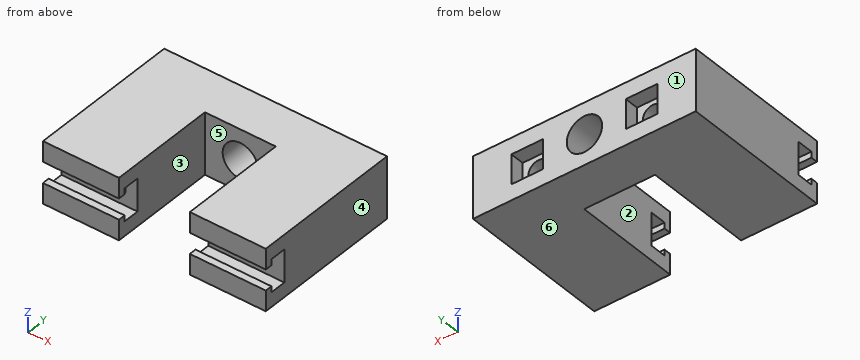
from build123d import *

# Parameters (mm, degrees)
F1_DEPTH = 11.049
F3_DEPTH = 39.9425
F4_R     = 3.175
F4_R_2   = 1.79705
F5_DEPTH = 27.307296
F4_W     = 5.678279
F4_H     = 5.299044
F6_DEPTH = 2.54


with BuildPart() as f1:
    # F0 (on Top) → F1 (new body)
    with BuildSketch(Plane.XY):
        Polygon((-17.543431, 48.29058), (-17.543431, 22.254284), (-3.922681, 22.254284), (-3.922681, 26.382432), (-3.922681, 41.622432), (8.777319, 41.622432), (8.777319, 26.382432), (8.777319, 22.254284), (22.398069, 22.254284), (22.398069, 48.29058), (22.398069, 49.56058), (-17.543431, 49.56058), align=None)
    extrude(amount=F1_DEPTH)

    # F2 (on face) → F3 (cut, through all)
    with BuildSketch(Plane(origin=(-17.543431, 0, 0), x_dir=(0, -1, 0), z_dir=(-1, 0, 0))):
        Polygon((-23.524284, 2.794), (-23.524284, 3.66395), (-22.254284, 3.66395), (-22.254284, 7.38505), (-23.524284, 7.38505), (-23.524284, 8.255), (-23.524284, 8.4455), (-26.419884, 8.4455), (-26.419884, 8.255), (-26.419884, 2.794), (-26.419884, 2.6035), (-23.524284, 2.6035), align=None)
    extrude(amount=-F3_DEPTH, mode=Mode.SUBTRACT)

    # F4 (on face) → F5 (cut, through all)
    with BuildSketch(Plane(origin=(0, 49.56058, 0), x_dir=(-1, 0, 0), z_dir=(0, 1, 0))):
        with Locations((-2.423196, 5.467734)):
            Circle(F4_R)
        with Locations((-12.678446, 5.467734)):
            Circle(F4_R_2)
        with Locations((7.832054, 5.467734)):
            Circle(F4_R_2)
    extrude(amount=-F5_DEPTH, mode=Mode.SUBTRACT)

    # F4 (on face) → F6 (cut)
    with BuildSketch(Plane(origin=(0, 49.56058, 0), x_dir=(-1, 0, 0), z_dir=(0, 1, 0))):
        with Locations((-12.678445, 5.467734)):
            Rectangle(F4_W, F4_H)
        with Locations((-12.678446, 5.467734)):
            Circle(F4_R_2, mode=Mode.SUBTRACT)
        with Locations((7.832054, 5.467734)):
            Rectangle(F4_W, F4_H)
        with Locations((7.832054, 5.467734)):
            Circle(F4_R_2, mode=Mode.SUBTRACT)
    extrude(amount=-F6_DEPTH, mode=Mode.SUBTRACT)


solid = f1.part
Verification items for the finished model (mm, model axes). Face numbers are marked on the shaded views. A direction names the side the tool comes from. Give positions to 0.01 mm unless a question says otherwise; leave off trailing zeros. Loops run counter-clockwise (first coordinate to the right, second up) from the corner with the lowest first, then second, coordinate; pieces in that order, holes last. Notation, with made-up numbers: (-29.5, 9.5) - (-9.5, 9.5) arc R11 ccw to (-9.5, 24.5) - close; hole circle Ø8 at (72, 82.25). An arc over 180 degrees is marked (long way). Write item = value, one per line. Start each with the question number.
Q1. Depth check by flat-ended pin: P1, Ø1, axis at x = 3, z = 9, coming from the -Y side. Enter the tip coordinate at first touch or a pass-through.
Q2. Cross-section at B-B, the plane y = 35.5. Enter the section's corners in (x, z), and give its area (3 significant figures).
Q3. Thickness scan on line 1 (X direction, y = 44, z = 5.5); line 2 (Y direction, x = 17.5, z = 7.5); line 3 (X direction, y = 33.25, z = 10.5). Record the ranges inside material, lowest first.
Q4. Cross-section at C-C, the plane z = 9.75. Enter the section's corners in (x, y), and give its area (3 significant figures).
Q5. Mould release check, pull along X, two halves, no side actions. Record for the marked faces 1, 2, 3 and 4: released by +X, released by -X, zero draft, split by the parting line, or undercut.
Q6. Cross-section at D-D, the plane x = 1. Enter the section's corners in (y, z).
Q7. Cross-section at A-A, the plane y = 24.25. Enter the section's corners in (x, z), and give its area (3 significant figures).
Q8. Tool access check on the marked faces 5 and 6. Record the directions out of +Z, -Z, +X, -X, +Y, -Y that give a thin tool (end or side, any length) a straight path to the whole face; none if there is none.
Answer key:
q1.P1 = 41.62
q2.outline = (-17.54, 0) - (-3.92, 0) - (-3.92, 11.05) - (-17.54, 11.05) - close; (8.78, 0) - (22.4, 0) - (22.4, 11.05) - (8.78, 11.05) - close; hole circle Ø3.59 at (-7.83, 5.47); hole circle Ø3.59 at (12.68, 5.47)
q2.area = 281 mm^2
q3.line_1 = -17.54 to -9.63, -6.04 to -0.75, 5.6 to 10.88, 14.48 to 22.4
q3.line_2 = 22.25 to 23.52, 26.42 to 49.56
q3.line_3 = -17.54 to -3.92, 8.78 to 22.4
q4.outline = (-17.54, 22.25) - (-3.92, 22.25) - (-3.92, 41.62) - (8.78, 41.62) - (8.78, 22.25) - (22.4, 22.25) - (22.4, 49.56) - (-17.54, 49.56) - close
q4.area = 845 mm^2
q5.face_1 = zero draft
q5.face_2 = undercut
q5.face_3 = undercut
q5.face_4 = released by +X
q6.outline = (41.62, 0) - (49.56, 0) - (49.56, 2.63) - (41.62, 2.63) - close; (41.62, 8.31) - (49.56, 8.31) - (49.56, 11.05) - (41.62, 11.05) - close
q7.outline = (-17.54, 0) - (-3.92, 0) - (-3.92, 2.6) - (-17.54, 2.6) - close; (-17.54, 8.45) - (-3.92, 8.45) - (-3.92, 11.05) - (-17.54, 11.05) - close; (8.78, 0) - (22.4, 0) - (22.4, 2.6) - (8.78, 2.6) - close; (8.78, 8.45) - (22.4, 8.45) - (22.4, 11.05) - (8.78, 11.05) - close
q7.area = 142 mm^2
q8.face_5 = +Z, -Z, -Y
q8.face_6 = -Z, +X, -X, +Y, -Y
